Source: CAD feature listing. Evaluate the final solid. Frame: model axes, mm. A direction names the side the tool comes from. Give positions to 0.01 mm unless a question says otherwise; leave off trailing zeros. Order: outer loops, then holes, each group sorted by start corner. A loop starts at its lowest first (then second) coordinate and runs counter-clockwise, first axis right, second up. Notation, with made-up numbers: M 42.25,80 L 63.25,80 A21 ccw 63.25,110 Z; hole C 7,6.5 d3. An arc over 180 degrees is marked long. Use CSV: the item, a comma, the result in double quotes. Start each with the question number.
Item 1: Pull-direction query (X, two-part tool) for faces 1 (the face through (21.57, -2.52, 0.9)), 2 (the face through (2.03, -2.66, 6.11)), 3 (the face through (-15.27, -10.098, 8.715)); classes: +X half, -X half, draft (parallel to the pull), parting line (faces both ways), or undercut.
Item 2: Section query C-C on y = -9.5. Return loops of the section in (x, z).
Item 3: Section query D-D on z = 4. Count the separate pieces of the cut face and the enclosed holes in it, and give its area (3 significant figures).
Item 4: Section query A-A on x = -10.5. Return loops of the section in (y, z), and give its area (3 significant figures).
Item 5: Ray query, probe 1 along X at (y, z) = (-10, 6.3); probe 2 along X at (y, z) = (-2.6, 4); probe 3 along X at (y, z) = (-15.25, 5.25). Return the intervals inside material, ascending. Write a range as from..to.
Item 6: Access query for faces 4 (the face through (-1.43, -19.715, 11.029)), 5 (the face through (-7.96, -11.49, 1.48)), 6 (the face through (3.633, -15.544, 2.095)), 7 (the face through (22.129, -0.285, 3.697)), 8 (the face through (-5, -10, 4)). Directions: +Z, -Z, +X, -X, +Y, -Y. A direction counts if a zero-diameter tool reaches every point of the face in a straight line with its end or side. Return the directions, or none.
Item 7: First-contact query: pin 1 (1.5 mm diameter, centred on y = -6, z = 4, fed in from +X); pin 2 (8 mm diameter, centred on y = -12, z = 12.5, fed in from -X); pin 3 (2 mm diameter, centred on x = 5, z = 5.5, fed in from -Y); pin 4 (7 mm diameter, centred on y = -8.5, z = 6, fed in from +X). Flat tips, straight axial feed; report the tip coordinate or a pass-through.
Item 8: Section query B-B on x = -6.5. Return loops of the section in (y, z), and give its area (3 significant figures).
from build123d import *

# Parameters (mm, degrees)
SKETCH012_R            = 2.4
SKETCH012_R_2          = 1.6
PAD010_DEPTH           = 30
CYLINDER005_R          = 4
CYLINDER005_DEPTH      = 5
CYLINDER005_ROLL_ANGLE = 90
CYLINDER004_R          = 4
CYLINDER004_DEPTH      = 5
CYLINDER004_ROLL_ANGLE = 90
CHAMFER_SIZE           = 0.5
CYLINDER003_R          = 1.7
CYLINDER003_DEPTH      = 15
PRISM_DEPTH            = 10
BOX013_W               = 30
BOX013_H               = 12
BOX013_DEPTH           = 20
PAD009_DEPTH           = 20
FILLET015_R            = 3
FILLET016_R            = 1


with BuildPart() as pad010:
    # Sketch012 → Pad010 (new body)
    with BuildSketch(Plane.XZ.offset(-5)):
        with Locations((4.42924, 6)):
            Circle(SKETCH012_R)
        with Locations((18.42924, 4)):
            Circle(SKETCH012_R_2)
    extrude(amount=PAD010_DEPTH)


with BuildPart() as cylinder005:
    # Cylinder005 → Cylinder005 (new body)
    with BuildSketch(Plane.XY):
        Circle(CYLINDER005_R)
    extrude(amount=CYLINDER005_DEPTH)


with BuildPart() as cylinder005_1:
    # Cylinder005 roll: moved
    add(cylinder005.part.rotate(Axis((0, 0, 0), (1, 0, 0)), CYLINDER005_ROLL_ANGLE))


with BuildPart() as cylinder005_2:
    # Cylinder005 placement: moved
    add(cylinder005_1.part.moved(Location((4.5, -14.6, 6))))


with BuildPart() as chamfer_body:
    # Cylinder004 → Cylinder004 (new body)
    with BuildSketch(Plane.XY):
        Circle(CYLINDER004_R)
    extrude(amount=CYLINDER004_DEPTH)


with BuildPart() as chamfer_body_1:
    # Cylinder004 roll: moved
    add(chamfer_body.part.rotate(Axis((0, 0, 0), (1, 0, 0)), CYLINDER004_ROLL_ANGLE))


with BuildPart() as chamfer_body_2:
    # Cylinder004 placement: moved
    add(chamfer_body_1.part.moved(Location((4.5, -0.4, 6))))

    # Fusion006: union Cylinder005
    add(cylinder005_2.part)

    # Chamfer
    chamfer_edges = [chamfer_body_2.edges().sort_by_distance(p)[0] for p in [
        (0.5, -5.4, 6),
        (0.5, -14.6, 6),
    ]]
    chamfer(chamfer_edges, length=CHAMFER_SIZE)


with BuildPart() as cylinder003:
    # Cylinder003 → Cylinder003 (new body)
    with BuildSketch(Plane(origin=(-10.5, -10, -2), x_dir=(1, 0, 0), z_dir=(0, 0, 1))):
        Circle(CYLINDER003_R)
    extrude(amount=CYLINDER003_DEPTH)


with BuildPart() as prism:
    # Prism → Prism (new body)
    with BuildSketch(Plane(origin=(-10.5, -10, -7), x_dir=(1, 0, 0), z_dir=(0, 0, 1))):
        Polygon((3.4, 0), (1.7, 2.944486), (-1.7, 2.944486), (-3.4, 0), (-1.7, -2.944486), (1.7, -2.944486), align=None)
    extrude(amount=PRISM_DEPTH)


with BuildPart() as cube013:
    # Box013 → Box013 (new body)
    with BuildSketch(Plane(origin=(-5, -16, -2), x_dir=(1, 0, 0), z_dir=(0, 0, 1))):
        with Locations((15, 6)):
            Rectangle(BOX013_W, BOX013_H)
    extrude(amount=BOX013_DEPTH)


with BuildPart() as cut021:
    # Sketch011 → Pad009 (new body)
    with BuildSketch(Plane.XZ):
        Polygon((-15.57076, 9), (-3.884468, 9), (1.115532, 14), (14.086094, 14), (22.42924, 5.656854), (22.42924, 0), (-15.57076, 0), align=None)
    extrude(amount=PAD009_DEPTH)

    # Cut018: cut Cube013
    add(cube013.part, mode=Mode.SUBTRACT)

    # Cut019: cut Prism
    add(prism.part, mode=Mode.SUBTRACT)

    # Cut020: cut Cylinder003
    add(cylinder003.part, mode=Mode.SUBTRACT)

    # Fillet015
    fillet015_edges = [cut021.edges().sort_by_distance(p)[0] for p in [
        (-15.57076, 0, 4.5),
        (-15.57076, -20, 4.5),
        (22.42924, -2, 5.656854),
        (22.42924, -2, 0),
        (22.42924, -18, 0),
        (22.42924, -18, 5.656854),
    ]]
    fillet(fillet015_edges, radius=FILLET015_R)

    # Fillet016
    fillet016_edges = [cut021.edges().sort_by_distance(p)[0] for p in [
        (-14.69208, -19.12132, 9),
        (-8.227614, -20, 9),
        (-1.384468, 0, 11.5),
        (7.600813, 0, 14),
        (17.818327, 0, 10.267767),
        (1.115532, -2, 14),
        (-1.384468, -20, 11.5),
        (7.600813, -20, 14),
        (17.818327, -20, 10.267767),
        (1.115532, -18, 14),
        (14.086094, -2, 14),
        (14.086094, -18, 14),
    ]]
    fillet(fillet016_edges, radius=FILLET016_R)

    # Fusion007: union Chamfer body
    add(chamfer_body_2.part)

    # Cut021: cut Pad010
    add(pad010.part, mode=Mode.SUBTRACT)


solid = cut021.part
Verdict:
1,face 1,"+X half"
1,face 2,"undercut"
1,face 3,"-X half"
2,outline,"M -15.57,1 A1 ccw -14.57,0 L -13.61,0 L -13.61,3 L -12.12,3 L -12.12,9 L -14.57,9 A1 ccw -15.57,8 Z; M -8.88,3 L -7.39,3 L -7.39,0 L -5,0 L -5,9 L -8.88,9 Z"
3,separate pieces,"5"
3,enclosed holes,"1"
3,area,"382 mm2"
4,outline,"M -20,1 A1 ccw -19,0 L -12.94,0 L -12.94,3 L -11.7,3 L -11.7,9 L -19,9 A1 ccw -20,8 Z; M -8.3,3 L -7.06,3 L -7.06,0 L -1,0 A1 ccw 0,1 L 0,8 A1 ccw -1,9 L -8.3,9 Z"
4,area,"141 mm2"
5,probe 1,"-15.57..-12.2, -8.8..-5"
5,probe 2,"-15.54..3.1, 5.76..16.83, 20.03..22.43"
5,probe 3,"-15.57..-5, 0.57..2.15, 6.71..8.43"
6,face 4,"+Z, -X, -Y"
6,face 5,"-Z"
6,face 6,"none"
6,face 7,"+Z, -Z, +X, +Y"
6,face 8,"+Z, -Z"
7,pin 1,"x = 7.66"
7,pin 2,"x = -15.44"
7,pin 3,"through"
7,pin 4,"x = 8.4"
8,outline,"M -20,1 A1 ccw -19,0 L -1,0 A1 ccw 0,1 L 0,8 A1 ccw -1,9 L -19,9 A1 ccw -20,8 Z"
8,area,"179 mm2"
